Work out the finished part from the listing and answer in its coordinate system (mm). Face numbers are marked on the shaded views. A direction names the side the tool comes from. Coordinates: 2 decimals unless noted, no trailing zeros. Order: outer loops, then holes, each group sorted by start corner. A loop starts at its lowest first (then second) coordinate and runs counter-clockwise, first axis right, second up.
1. The part is cut by section A-A, the plane x = 2.25. Give the vertices of the cut face in (y, z).
2. Flat-ended cylindrical pins translate along their axes: pin 1 Ø2 at (x, y) = (-5, 12.5) entering from -Z; pin 2 Ø3 at (x, z) = (7.5, 11) entering from -Y; pin 3 Ø1 at (x, y) = (3, -11) entering from +Z; pin 4 Ø2 at (x, y) = (-6.5, 4.5) entering from -Z. Find the tip coordinate at first contact, or state that the pin passes through.
3. The part is cut by section B-B, the plane z = 4.25. Give the vertices of the cut face in (x, y), then the cut area to 3 significant figures.
4. A tool of negligible diameter and unlimited length cuts with its end or side. For the marked faces 1 and 2, from which of +Z, -Z, +X, -X, +Y, -Y can it reach the whole face along a straight path? Write none if from no direction.
5. Find the intervals of material crossed by probe 1 along Z at (x, y) = (6.5, 6.5); probe 2 along Y at (x, z) = (7.25, 5); probe 3 along X at (y, z) = (-2.5, 3), in increasing order.
```python
from build123d import *

# Parameters (mm, degrees)
DODANIE_WYCI_GNI_CIE1_DEPTH     = 20
WYTNIJ_WYCI_GNI_CIE2_DEPTH      = 10
WYTNIJ_WYCI_GNI_CIE2_DEPTH_BACK = 10
WYTNIJ_WYCI_GNI_CIE3_DEPTH      = 40


with BuildPart() as part:
    # Szkic2 → Dodanie-wyci_gni_cie1 (new body)
    with BuildSketch(Plane.XY):
        Polygon((0, 20), (-10, 0), (0, -20), (10, 0), align=None)
    extrude(amount=DODANIE_WYCI_GNI_CIE1_DEPTH)

    # Szkic6 → Wytnij-wyci_gni_cie2 (cut, two sides)
    with BuildSketch(Plane(origin=(0, 0, 0), x_dir=(0, 0, -1), z_dir=(1, 0, 0))) as wytnij_wyci_gni_cie2_sk:
        Polygon((-20, 0), (-20, 20), (0, 20), (0, -20), (-20, -20), align=None)
        Polygon((-10, 19.9), (-19.9, 0), (-10, -19.9), (-0.1, 0), align=None, mode=Mode.SUBTRACT)
    extrude(amount=WYTNIJ_WYCI_GNI_CIE2_DEPTH, mode=Mode.SUBTRACT)
    extrude(wytnij_wyci_gni_cie2_sk.sketch, amount=-WYTNIJ_WYCI_GNI_CIE2_DEPTH_BACK, mode=Mode.SUBTRACT)

    # Szkic7 → Wytnij-wyci_gni_cie3 (cut)
    with BuildSketch(Plane(origin=(-5.024810608, 0, 5.05018844), x_dir=(-0.708885658, 0, -0.705323418), z_dir=(0.705323418, 0, -0.708885658))):
        Polygon((7.018324235, 0), (-7.017789899, 19.9), (-21.1247926, 0), (-7.088678465, -19.9), align=None)
    extrude(amount=-WYTNIJ_WYCI_GNI_CIE3_DEPTH, mode=Mode.SUBTRACT)


solid = part.part
```
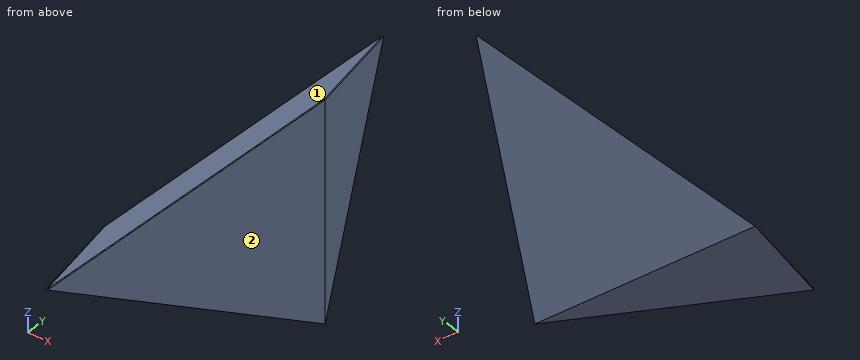
Geometry says:
1. outline: (-15.5, 7.81) - (0, 0.1) - (15.5, 7.81) - (15.5, 12.19) - (15.3, 12.29) - (-15.3, 12.29) - (-15.5, 12.19) - close
2. pin 1: passes through
2. pin 2: stops at y = -8
2. pin 3: stops at z = 13.53
2. pin 4: stops at z = 1.84
3. outline: (-5.87, -8.26) - (-5.83, -8.34) - (5.83, -8.34) - (10, 0) - (5.83, 8.34) - (-5.83, 8.34) - (-5.83, -8.3) - close
3. area: 229 mm2
4. face 1: +Z, -X, +Y
4. face 2: +Z, -Z, +X, -Y
5. probe 1: z = 3.33 to 16.52
5. probe 2: y = -5.5 to 5.5
5. probe 3: x = -7.09 to 8.75
